Part model, mm, in its own coordinate system. A direction names the side the tool comes from. Coordinates: 2 decimals unless noted, no trailing zeros. Order: outer loops, then holes, each group sorted by start corner. A loop starts at its lowest first (then second) coordinate and runs counter-clockwise, first axis right, second up.
Autodesk Inventor part; units mm, degrees
ref_plane "Plano de trabajo1" through (0, 14.2, 0) normal (0, 1, 0) x (1, 0, 0)
ref_plane "YZ Plane" through (0, 0, 0) normal (1, 0, 0) x (0, 1, 0)
ref_plane "XZ Plane" through (0, 0, 0) normal (0, 1, 0) x (-1, 0, 0)
sketch "Boceto1" plane through (0, 0, 0) normal (0, 1, 0) x (-1, 0, 0)
  circle A0 centre (0, 0) radius 26
  dimension "d0" = 52
extrude "Extrusión1" add sketch "Boceto1" along normal blind 4
sketch "Boceto2" plane through (0, 4, 0) normal (0, 1, 0) x (1, 0, 0)
  circle A0 centre (0, 0) radius 21.775
  dimension "d3" = 43.55
extrude "Extrusión2" add sketch "Boceto2" along normal blind 13.8
ref_plane "Plano de trabajo1" through (0, 14.2, 0) normal (0, 1, 0) x (1, 0, 0)
sketch "Boceto6" plane through (0, 14.2, 0) normal (0, 1, 0) x (1, 0, 0)
  circle A0 centre (0, 0) radius 21.775
  circle A1 centre (0, 0) radius 18.925
  dimension "d18" = 37.85
extrude "Extrusión6" cut sketch "Boceto6" against normal blind 5
sketch "Boceto7" plane through (0, 0, 0) normal (0, -1, 0) x (1, 0, 0)
  circle A0 centre (0, 0) radius 18.925
  circle A1 centre (0, 0) radius 21.775
  circle A2 centre (0, 0) radius 26
  line L0 (0, 26) -> (0, 20.5)
  line L1 (0, 20.5) -> (0, 3.45)
  arc A3 (8.0792, 17.1138) -> (4.3595, 20.5) centre (0, 11.975) ccw
  line L2 (0, 3.45) -> (4.3595, 3.45)
  line L3 (0, 3.45) -> (-4.3595, 3.45)
  line L4 (0, 20.5) -> (4.3595, 20.5)
  line L5 (0, 20.5) -> (-4.3595, 20.5)
  arc A4 (4.3595, 3.45) -> (8.0792, 17.1138) centre (0, 11.975) ccw
  arc A5 (-4.3595, 3.45) -> (4.3595, 3.45) centre (0, 11.975) ccw
  arc A6 (4.3595, 20.5) -> (-4.3595, 20.5) centre (0, 11.975) ccw
  arc A7 (-4.3595, 20.5) -> (-4.3595, 3.45) centre (0, 11.975) ccw
  dimension "d21" = 5.5
  dimension "d22" = 17.05
  dimension "d23" = 19.15
extrude "Extrusión7" cut sketch "Boceto7" against normal blind 4.45 contours A4 L2 L1 A0 | A0 L1 L4 A3 | A7 L5 L1 A0 | A0 L1 L3 A7
sketch "Boceto8" plane through (0, 4.45, 0) normal (0, -1, 0) x (1, 0, 0)
  arc A0 (-4.3595, 20.5) -> (-4.3595, 3.45) centre (0, 11.975) ccw
  circle A1 centre (0, 11.975) radius 5.275
  point P0 (0, 0)
  dimension "d26" = 10.55
extrude "Extrusión8" cut sketch "Boceto8" against normal blind 15
sketch "Boceto9" plane through (0, 0, 0) normal (0, -1, 0) x (1, 0, 0)
  line L0 (4.3595, 3.45) -> (-4.3595, 3.45)
  line L1 (0, 3.45) -> (0, 2.45)
  line L2 (0, 2.45) -> (0, -20.8)
  circle A0 centre (0, -9.175) radius 11.625
  point P0 (0, 0)
  dimension "d29" = 1
  dimension "d30" = 23.25
extrude "Extrusión9" cut sketch "Boceto9" against normal blind 4.25
sketch "Boceto10" plane through (0, 4.25, -9.175) normal (0, -1, 0) x (1, 0, 0)
  circle A0 centre (0, 0) radius 7.275
  point P0 (0, 9.175)
  dimension "d33" = 14.55
extrude "Extrusión10" cut sketch "Boceto10" against normal up to surface (13.55 mm away)
thread "Rosca2"
sketch "Boceto11" plane through (0, 17.8, 0) normal (0, 1, 0) x (1, 0, 0)
  line L0 (0, 0) -> (-13.15, 0)
  line L1 (0, 0) -> (13.15, 0)
  circle A0 centre (-13.15, 0) radius 1
  circle A1 centre (13.15, 0) radius 1
  dimension "d38" = 13.15
  dimension "d39" = 13.15
  dimension "d40" = 2
  dimension "d41" = 2
extrude "Extrusión11" cut sketch "Boceto11" against normal blind 5
properties part number "Pieza_sonar"
(1) Pull direction X, two halves, no side cores. Call faces 5 (the face through (0, 17.8, 0)), 6 (the face through (6.472, 2.194, 19.031)), 7 (the face through (-4.72, 6.564, -21.257)): +X half, -X half, draft (parallel to the pull), parting line (faces both ways), or undercut.
(2) Slice it at A-A, the plane x = 0. State how many separate pieces and enclosed holes the cut face has, then the cut area to 3 significant figures.
(3) Tool access for faces 1 (the face through (-7, 14.2, -18)), 2 (the face through (-13, 12.8, 0)), 3 (the face through (6.25, 2.095, 0.627)), 4 (the face through (-3.89, 11.03, 15.54)): list every direction of +Z, -Z, +X, -X, +Y, -Y with a clear straight run to the whole face (end or side of a thin tool).
(4) Slice it at B-B, the plane z = -10. Give the cut face in (x, y), then the cut area to 3 significant figures.
(5) Slice it at D-D, the plane z = 18. Give the cut face in (x, y), then the cut area to 3 significant figures.
(6) Drop flat-ended pins along their axis: pin 1 (1.5 mm diameter, centred on y = 3.5, z = 15, fed in from +X); pin 2 (1.6 mm diameter, centred on x = 13.15, z = 0, fed in from -Y); pin 3 (5 mm diameter, centred on y = 12, z = 13.5, fed in from -X); pin 4 (2 mm diameter, centred on y = 6, z = -14, fed in from -X). Give the stop position or say it passes through.
(7) Probe line 1 (Z direction, x = 0, y = 2.4); line 2 (X direction, y = 13.8, z = 0) (3 decimals); line 3 (Y direction, x = 9.5, z = 17). List the from-to ranges inside material, lowest first.
(8) Slice it at C-C, the plane x = 21. Give the cut face in (y, z), then the cut area to 3 significant figures.
Here are the results:
1. face 5: draft
1. face 6: undercut
1. face 7: parting line
2. separate pieces: 3
2. enclosed holes: 0
2. area: 268 mm2
3. face 1: none
3. face 2: +Y
3. face 3: -Y
3. face 4: +Y, -Y
4. outline: (-24, 0) - (-11.6, 0) - (-11.6, 4.25) - (-7.23, 4.25) - (-7.23, 17.8) - (-19.34, 17.8) - (-19.34, 14.2) - (-16.07, 14.2) - (-16.07, 9.2) - (-19.34, 9.2) - (-19.34, 4) - (-24, 4) - close; (7.23, 4.25) - (11.6, 4.25) - (11.6, 0) - (24, 0) - (24, 4) - (19.34, 4) - (19.34, 9.2) - (16.07, 9.2) - (16.07, 14.2) - (19.34, 14.2) - (19.34, 17.8) - (7.23, 17.8) - close
4. area: 399 mm2
5. outline: (-18.76, 0) - (-7.44, 0) - (-7.44, 4.45) - (7.44, 4.45) - (7.44, 0) - (18.76, 0) - (18.76, 4) - (12.25, 4) - (12.25, 9.2) - (5.84, 9.2) - (5.84, 14.2) - (12.25, 14.2) - (12.25, 17.8) - (-12.25, 17.8) - (-12.25, 14.2) - (-5.84, 14.2) - (-5.84, 9.2) - (-12.25, 9.2) - (-12.25, 4) - (-18.76, 4) - close
5. area: 358 mm2
6. pin 1: stops at x = 21.75
6. pin 2: stops at y = 0
6. pin 3: stops at x = -17.96
6. pin 4: stops at x = -17.47
7. line 1: z = -26 to -20.8, 2.45 to 3.45, 20.5 to 26
7. line 2: x = -18.925 to -14.15, -12.15 to 12.15, 14.15 to 18.925
7. line 3: y = 0 to 9.2, 14.2 to 17.8
8. outline: (0, -15.33) - (4, -15.33) - (4, -5.76) - (9.2, -5.76) - (9.2, 5.76) - (4, 5.76) - (4, 15.33) - (0, 15.33) - close; (14.2, -5.76) - (17.8, -5.76) - (17.8, 5.76) - (14.2, 5.76) - close
8. area: 224 mm2
